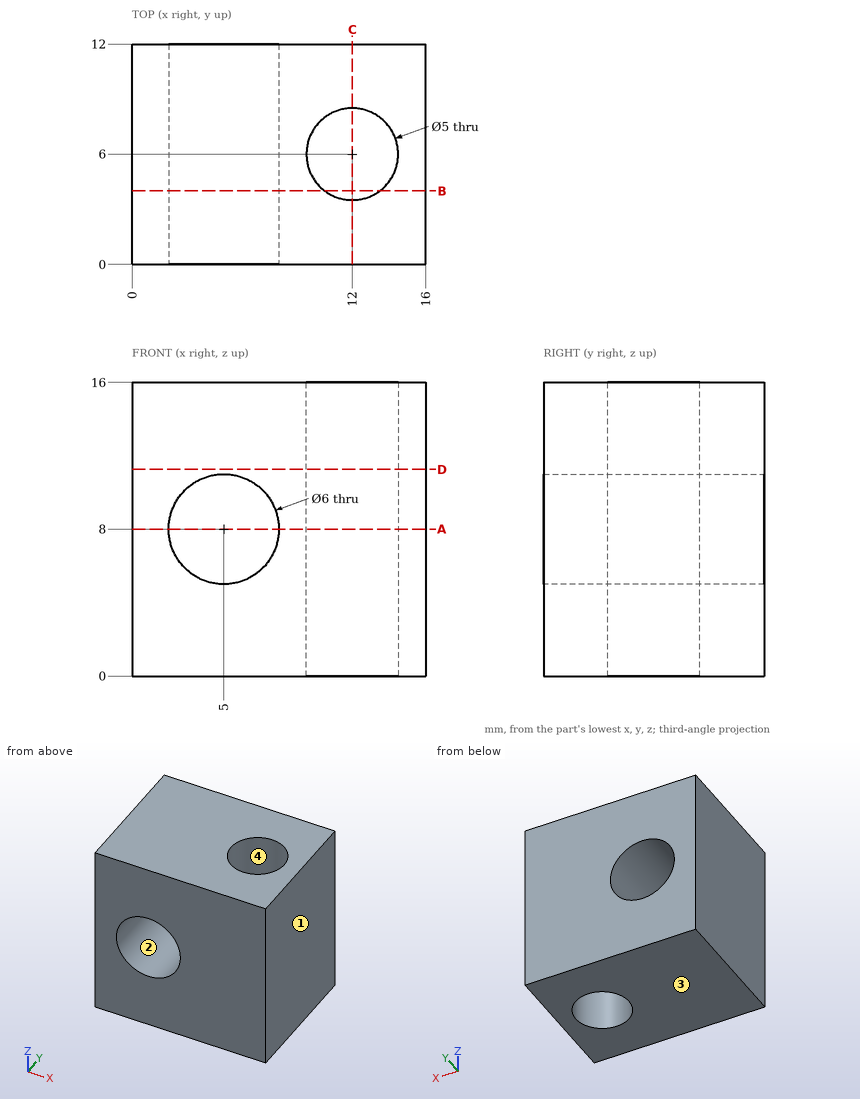
The figure shows three views and two pictorial views of one solid part (mm, origin at its lowest corner). Answer the questions. Round coordinates to 2 decimals unless told otherwise and drop trailing zeros. Order: outer loops, then holes, each group sorted by start corner. A loop starts at its lowest first (then second) coordinate and runs counter-clockwise, first axis right, second up. Notation, with made-up numbers: (46, 83.5) - (51, 83.5) arc R30 ccw to (51, 113.5) - close; hole circle Ø2 at (-32.75, 4.5). An arc over 180 degrees is marked (long way). Write item = value, one per line. Start each with the question number.
1) Section D-D, the plane z = 11.25 is taken. Write down the section's boundary in (x, y), plus the area to 3 significant figures.
2) Given pin 1 (4 mm diameter, centred on x = 12, y = 6, fed in from +Z), flat-ended and moving along its own axis, determine where the tip first touches the part or whether it passes through.
3) Section B-B, the plane y = 4 is taken. Write down the section's boundary in (x, z).
4) For a pull along X with two mould halves and no side action, classify the marked faces 1, 2, 3 and 4 as released by +X, released by -X, zero draft, split by the parting line, or undercut.
5) Straight lines are drawn through the part: L1, parallel to Y at x = 12, z = 5.25; L2, parallel to X at y = 2.75, z = 8; L3, parallel to X at y = 7.75, z = 3.25. For each, find the intervals that lie inside material, in ascending order.
6) Section A-A, the plane z = 8 is taken. Write down the section's boundary in (x, y), plus the area to 3 significant figures.
7) Section C-C, the plane x = 12 is taken. Write down the section's boundary in (y, z), plus the area to 3 significant figures.
Results list:
q1.outline = (0, 0) - (16, 0) - (16, 12) - (0, 12) - close; hole circle Ø5 at (12, 6)
q1.area = 172 mm^2
q2.pin_1 = through
q3.outline = (0, 0) - (10.5, 0) - (10.5, 16) - (0, 16) - close; (13.5, 0) - (16, 0) - (16, 16) - (13.5, 16) - close; hole circle Ø6 at (5, 8)
q4.face_1 = released by +X
q4.face_2 = undercut
q4.face_3 = zero draft
q4.face_4 = undercut
q5.L1 = 0 to 3.5, 8.5 to 12
q5.L2 = 0 to 2, 8 to 16
q5.L3 = 0 to 10.21, 13.79 to 16
q6.outline = (0, 0) - (2, 0) - (2, 12) - (0, 12) - close; (8, 0) - (16, 0) - (16, 12) - (8, 12) - close; hole circle Ø5 at (12, 6)
q6.area = 100 mm^2
q7.outline = (0, 0) - (3.5, 0) - (3.5, 16) - (0, 16) - close; (8.5, 0) - (12, 0) - (12, 16) - (8.5, 16) - close
q7.area = 112 mm^2
